For this review, take the finished solid that the model builds, in its own axes (mm). A direction names the side the tool comes from. Give positions to 0.01 mm unless a question says otherwise; leave off trailing zeros. Write each loop counter-clockwise with the first axis right and the second up, starting at its lowest first coordinate (ties: lowest second). Pieces come first, ordered by that corner, then holes. Notation, with made-up numbers: (54.25, 88.25) -> (83.25, 88.25) arc R25 ccw to (83.25, 104.25) -> close; hole circle Ø6 at (-19, -30). An arc over 180 degrees is marked (long way). Write item = value, one per line.
```python
from build123d import *

# Parameters (mm, degrees)
SKETCH1_R               = 11.75
BOSS_EXTRUDE1_DEPTH     = 1.5
BOSS_EXTRUDE2_START     = 0.5
SKETCH2_R               = 3.5
BOSS_EXTRUDE2_DEPTH     = 4.3
CUT_EXTRUDE1_DEPTH      = 18.164352595
CUT_EXTRUDE1_DEPTH_BACK = 18.164352595
SKETCH3_R               = 1.25
SKETCH4_R               = 0.5
CUT_EXTRUDE2_DEPTH      = 18.045967265
SKETCH5_R               = 0.5
CUT_EXTRUDE3_DEPTH      = 17.77542846
CIRPATTERN1_COUNT       = 2
SKETCH6_R               = 2.375
CUT_EXTRUDE4_DEPTH      = 2.25


with BuildPart() as part:
    # Sketch1 → Boss-Extrude1 (new body)
    with BuildSketch(Plane(origin=(0, 0, 0), x_dir=(1, 0, 0), z_dir=(0, 1, 0))):
        with Locations(Location((0, 0, 0), (0, 0, 270))):
            Circle(SKETCH1_R)
    extrude(amount=BOSS_EXTRUDE1_DEPTH)

    # Sketch2 → Boss-Extrude2 (add)
    with BuildSketch(Plane(origin=(0, 1.5, 0), x_dir=(1, 0, 0), z_dir=(0, 1, 0)).offset(BOSS_EXTRUDE2_START)):
        with Locations(Location((0, 0, 0), (0, 0, 270))):
            Circle(SKETCH2_R)
    extrude(amount=-BOSS_EXTRUDE2_DEPTH)

    # Sketch3 → Cut-Extrude1 (cut, two sides: drawn at the far end of the back side and taken through both)
    with BuildSketch(Plane(origin=(0, 2, 0), x_dir=(1, 0, 0), z_dir=(0, 1, 0)).offset(-CUT_EXTRUDE1_DEPTH_BACK)):
        with Locations(Location((0, 0, 0), (0, 0, 270))):
            Circle(SKETCH3_R)
    extrude(amount=CUT_EXTRUDE1_DEPTH + CUT_EXTRUDE1_DEPTH_BACK, mode=Mode.SUBTRACT)

    # Sketch4 → Cut-Extrude2 (cut, through all)
    with BuildSketch(Plane(origin=(0, 1.5, 0), x_dir=(1, 0, 0), z_dir=(0, 1, 0))):
        with Locations(Location((9.75, 0, 0), (0, 0, 270))):
            Circle(SKETCH4_R)
        with Locations(Location((9.121794872, 3.443161094, 0), (0, 0, 270))):
            Circle(SKETCH4_R)
        with Locations(Location((9.121794872, -3.443161094, 0), (0, 0, 270))):
            Circle(SKETCH4_R)
    cut_extrude2 = extrude(amount=-CUT_EXTRUDE2_DEPTH, mode=Mode.SUBTRACT)

    # Sketch5 → Cut-Extrude3 (cut, symmetric)
    with BuildSketch(Plane(origin=(0, 0, 0), x_dir=(1, 0, 0), z_dir=(0, 1, 0))):
        with Locations(Location((0, 8, 0), (0, 0, 270))):
            Circle(SKETCH5_R)
        with Locations(Location((0, 10, 0), (0, 0, 270))):
            Circle(SKETCH5_R)
        with Locations(Location((3.445989517, 9.3875, 0), (0, 0, 270))):
            Circle(SKETCH5_R)
        with Locations(Location((2.756791613, 7.51, 0), (0, 0, 270))):
            Circle(SKETCH5_R)
        with Locations(Location((-2.756791613, 7.51, 0), (0, 0, 270))):
            Circle(SKETCH5_R)
        with Locations(Location((-3.445989517, 9.3875, 0), (0, 0, 270))):
            Circle(SKETCH5_R)
    cut_extrude3 = extrude(amount=CUT_EXTRUDE3_DEPTH, both=True, mode=Mode.SUBTRACT)

    # CirPattern1: Cut-Extrude2, Cut-Extrude3 ×2 about axis
    cirpattern1_axis = Axis((0, 0, 0), (0, 1, 0))
    add([cut_extrude2.rotate(cirpattern1_axis, i * 360 / CIRPATTERN1_COUNT) for i in range(1, CIRPATTERN1_COUNT)], mode=Mode.SUBTRACT)
    add([cut_extrude3.rotate(cirpattern1_axis, i * 360 / CIRPATTERN1_COUNT) for i in range(1, CIRPATTERN1_COUNT)], mode=Mode.SUBTRACT)

    # Sketch6 → Cut-Extrude4 (cut)
    with BuildSketch(Plane.XZ.offset(2.3)):
        with Locations(Location((0, 0, 0), (0, 0, 270))):
            Circle(SKETCH6_R)
    extrude(amount=-CUT_EXTRUDE4_DEPTH, mode=Mode.SUBTRACT)


solid = part.part
```
(1) Tool access review of faces 1 (the face through (-8.634, 0.76, -3.335)), 2 (the face through (-1.45, -1.19, 1.88)): name each direction out of +Z, -Z, +X, -X, +Y, -Y from which nothing blocks a thin tool from reaching the whole face with its end or side.
Answers below:
face_1 = +Y, -Y
face_2 = -Y
(2) For pin 1 (1.5 mm diameter, centred on y = 0, z = 1.5, fed in from +X); pin 2 (1.5 mm diameter, centred on x = 4, z = -8.5, fed in from +Y); pin 3 (3 mm diameter, centred on x = 0, z = 0, fed in from -Y), all flat-tipped, find the tip position at first contact; note any pin that passes through.
Answers below:
pin_1 = 11.73
pin_2 = 1.5
pin_3 = -0.05
(3) Take a section at C-C (x = -6.5). Write out the cut boundary in (y, z), plus the area to 3 significant figures.
Answers below:
outline = (0, -9.79) -> (1.5, -9.79) -> (1.5, 9.79) -> (0, 9.79) -> close
area = 29.4 mm^2
(4) Take a section at A-A (y = -1.45). Write out the cut boundary in (x, z) (3 decimals).
Answers below:
outline = circle Ø7 at (0, 0); hole circle Ø4.75 at (0, 0)
(5) The part is to be moulded in two halves that separate along Z. For faces 3 (the face through (0, 2, 2)), 4 (the face through (-3.417, -1.134, -0.759)), 5 (the face through (-9.306, 0.76, -0.231)), say which applies: released by +Z, released by -Z, zero draft, split by the parting line, or undercut.
Answers below:
face_3 = zero draft
face_4 = split by the parting line
face_5 = undercut
(6) Take a section at B-B (z = -5.5). Write out the cut boundary in (x, y).
Answers below:
outline = (-10.38, 0) -> (10.38, 0) -> (10.38, 1.5) -> (-10.38, 1.5) -> close
(7) To check wall thickness, follow probe 1 along X at (y, z) = (0.45, 0); probe 2 along Y at (x, z) = (-2, -10); probe 3 along X at (y, z) = (1.75, 0.25). State the ranges of each line that lie inside material, in increasing order.
Answers below:
probe_1 = -11.75 to -10.25, -9.25 to -1.25, 1.25 to 9.25, 10.25 to 11.75
probe_2 = 0 to 1.5
probe_3 = -3.49 to -1.22, 1.22 to 3.49
